```python
from build123d import *

# Parameters (mm, degrees)
F0_R        = 44.7584797017
F1_DEPTH    = 76.2
F2_DEPTH    = 25.4
F4_R        = 12.7
F3_W        = 25.4
F3_H        = 50.8
F5_DEPTH    = 25.4
F6_R        = 7.62
F7_T        = 2.54
F7_T3_DEPTH = 30.48
F7_T5_DEPTH = 55.88


# Not quite as in the source:
# - a shell that OpenCascade refuses in one call is made with other operations: the cavity is built on its own and cut out


with BuildPart() as f1:
    # F0 (on Front) → F1 (new body)
    with BuildSketch(Plane.XZ):
        Circle(F0_R)
    extrude(amount=F1_DEPTH)

    # F0 (on Front) → F2 (join)
    with BuildSketch(Plane.XZ):
        Circle(F0_R)
    extrude(amount=F2_DEPTH)

    # F4
    f4_edges = [f1.edges().sort_by_distance(p)[0] for p in [
        (-44.75848, 0, 0),
    ]]
    fillet(f4_edges, radius=F4_R)

    # F3 (on face) → F5 (join)
    with BuildSketch(Plane(origin=(0, 0, 0), x_dir=(-1, 0, 0), z_dir=(0, 1, 0))):
        Rectangle(F3_W, F3_H)
    extrude(amount=F5_DEPTH)

    # F6
    f6_edges = [f1.edges().sort_by_distance(p)[0] for p in [
        (-12.7, 25.4, 0),
        (0, 25.4, 25.4),
        (12.7, 25.4, 0),
        (0, 25.4, -25.4),
    ]]
    fillet(f6_edges, radius=F6_R)

    # F7: shell of thickness 2.54, made by hand


with BuildPart() as f7_core1:
    # F7_t2: copy of F1
    add(f1.part)

    # the walls: a layer under each face that stays
    f7_faces = [f7_core1.faces().sort_by_distance(p)[0] for p in [
        (0, 8.89, -25.4),
        (12.7, 8.89, 0),
        (0, 23.1681536726, -23.1681536726),
        (-21.3723198011, 0, -21.3723198011),
        (-12.7, 8.89, 0),
        (0, 8.89, 25.4),
        (10.4681536726, 23.1681536726, 0),
        (0, 25.4, 0),
        (-10.4681536726, 23.1681536726, 0),
        (-41.0387358228, -3.7197438789, 0),
        (0, 23.1681536726, 23.1681536726),
        (-44.7584797017, -44.45, 0),
    ]]
    thicken(f7_faces, amount=-F7_T, mode=Mode.SUBTRACT)

    # F7_s4 → F7_t3 (cut)
    with BuildSketch(Plane.YZ.offset(-15.24)):
        Polygon((0.0254, -25.4254), (0, -22.86), (-2.54, -22.86), (-2.54, -25.4), align=None)
        Polygon((0.0254, 25.4254), (-2.54, 25.4), (-2.54, 22.86), (0, 22.86), align=None)
    extrude(amount=F7_T3_DEPTH, mode=Mode.SUBTRACT)

    # F7_s6 → F7_t5 (cut)
    with BuildSketch(Plane.XY.offset(-27.94)):
        Polygon((12.7254, 0.0254), (10.16, 0), (10.16, -2.54), (12.7, -2.54), align=None)
        Polygon((-12.7254, 0.0254), (-12.7, -2.54), (-10.16, -2.54), (-10.16, 0), align=None)
    extrude(amount=F7_T5_DEPTH, mode=Mode.SUBTRACT)


with BuildPart() as f1_1:
    add(f1.part)

    # what is left inside the walls is the cavity
    f7_cavity = [f7_core1.part.solids().sort_by_distance(p)[0] for p in [
        (-42.19308, -55.033333, 0),
    ]]
    add(f7_cavity, mode=Mode.SUBTRACT)

    # F8: F1 across face


with BuildPart() as f1_2:
    add(f1_1.part)
    add(f1_1.part.mirror(Plane.XZ.offset(76.2)))


solid = f1_2.part
```
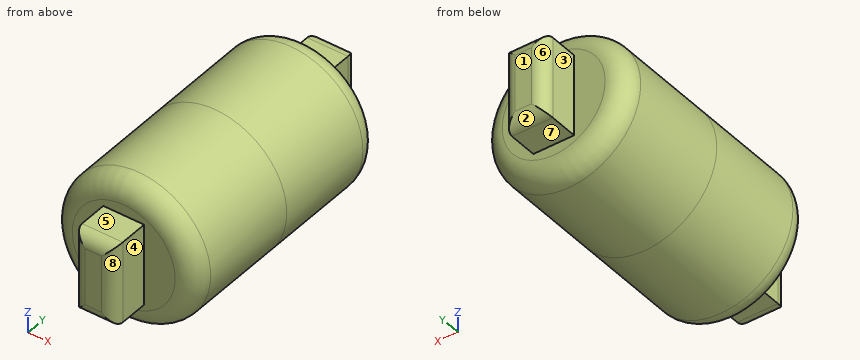
Work out the finished part from the listing and answer in its coordinate system (mm). Face numbers are marked on the shaded views. A direction names the side the tool comes from. Round coordinates to 2 decimals unless told otherwise and drop trailing zeros. Write each loop counter-clockwise with the first axis right and the second up, starting at its lowest first coordinate (ties: lowest second). Pieces come first, ordered by that corner, then holes.
1) A cutting plane is placed at A-A on y = 10.5. Determine the outline of the cut face in (x, z).
2) Flat-ended cylindrical pins translate along their axes: P1, Ø22.5, axis at y = 12.5, z = -3, coming from the -X side; P2, Ø5.5, axis at x = -1.5, y = 10.5, coming from the -Z side; P3, Ø10, axis at x = 4, y = -161.5, coming from the +Z side. Find the tip coordinate at first contact, or state that the pin passes through.
3) A cutting plane is placed at C-C on y = -144. Determine the outline of the cut face in (x, z), and give its area (3 significant figures).
4) Determine the mould class of the marked faces 6, 7 and 8 for opening direction Y: pulls with the +Y half, pulls with the -Y half, needs draft (parallel to the pull), parting line crosses it, or undercut.
5) A cutting plane is placed at B-B on y = -62.5. Determine the outline of the cut face in (x, z), and give its area (3 significant figures).
6) Which of the six approach directions +Z, -Z, +X, -X, +Y, -Y give full straight-line access (tool end or side, diameter ignored) to the marked faces 1, 2, 3, 4 and 5?
7) Consider probe 1 along Z at (x, y) = (0, -86); probe 2 along Y at (x, z) = (-18, 14); probe 3 along Z at (x, y) = (1.5, -21.5). Determine where each line is inside the solid, lowest interval first.
Entries:
1. outline: (-12.7, -25.4) - (12.7, -25.4) - (12.7, 25.4) - (-12.7, 25.4) - close; hole (-10.16, -22.86) - (10.16, -22.86) - (10.16, 22.86) - (-10.16, 22.86) - close
2. P1: stops at x = -12.7
2. P2: stops at z = -25.4
2. P3: stops at z = 25.4
3. outline: circle Ø88.02 at (0, 0); hole circle Ø82.53 at (0, 0)
3. area: 735 mm2
4. face 6: pulls with the +Y half
4. face 7: needs draft
4. face 8: pulls with the -Y half
5. outline: circle Ø89.52 at (0, 0); hole circle Ø84.44 at (0, 0)
5. area: 694 mm2
6. face 1: +Z, -Z, +X, -X, +Y
6. face 2: -Z, +X, -X, +Y
6. face 3: +Z, -Z, -X, +Y
6. face 4: +Z, -Z, +X, -Y
6. face 5: +Z, +X, -X, -Y
7. probe 1: z = -44.76 to -42.22, 42.22 to 44.76
7. probe 2: y = -152.4 to -149.86, -2.54 to 0
7. probe 3: z = -44.73 to -42.19, 42.19 to 44.73
